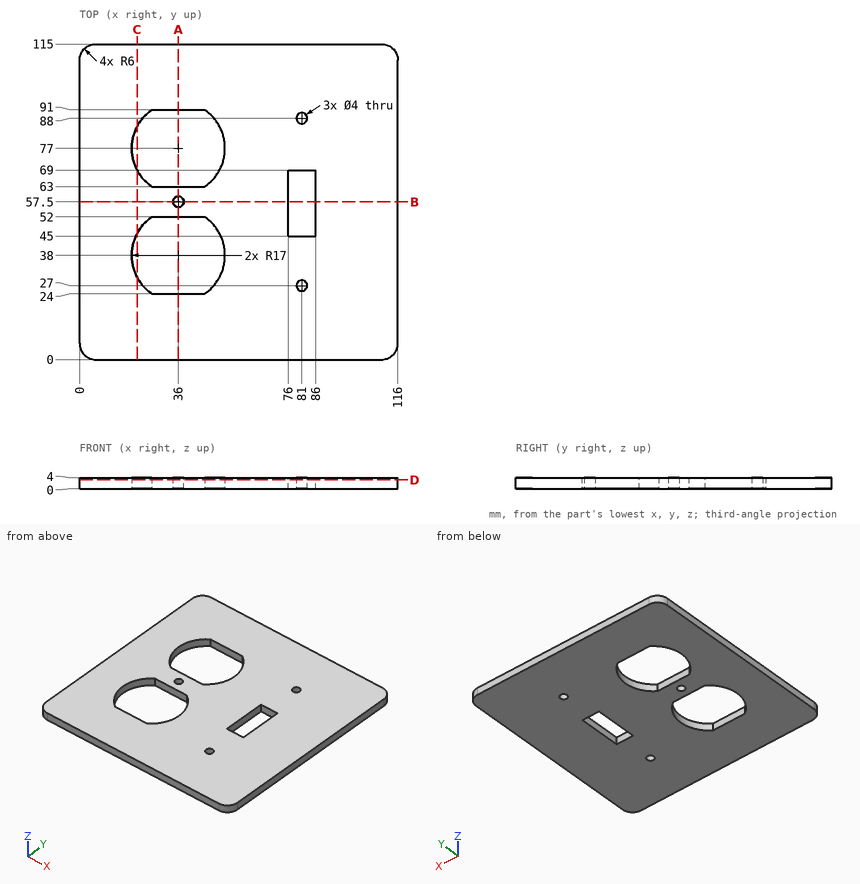
Design review of the part shown in the three views and the two pictorial views. Dimensions are in mm from the part's minimum x, y and z. Round coordinates to 2 decimals unless told otherwise and drop trailing zeros. Loops run counter-clockwise (first coordinate to the right, second up) from the corner with the lowest first, then second, coordinate; pieces in that order, holes last. Notation, with made-up numbers: M -6.5,3.25 L 42.5,3.25 A21 cw 42.5,26.25 Z; hole C -31,83.25 d8. An arc over 180 degrees is marked long. Put each result on its own line as item: value.
Q1. Consider section C-C, the plane x = 21. Give the boundary of the cut face in (y, z).
Result set:
outline: M 0,0 L 30,0 L 30,4 L 0,4 Z; M 46,0 L 69,0 L 69,4 L 46,4 Z; M 85,0 L 115,0 L 115,4 L 85,4 Z
Q2. Consider section D-D, the plane z = 3.2. Give the boundary of the cut face in (x, y), then the cut area to 3 significant figures.
Result set:
outline: M 0,6 A6 ccw 6,0 L 110,0 A6 ccw 116,6 L 116,109 A6 ccw 110,115 L 6,115 A6 ccw 0,109 Z; hole M 26.36,24 L 45.64,24 A17 ccw 45.64,52 L 26.36,52 A17 ccw Z; hole M 26.36,63 L 45.64,63 A17 ccw 45.64,91 L 26.36,91 A17 ccw Z; hole C 36,57.5 d4; hole M 76,45 L 86,45 L 86,69 L 76,69 Z; hole C 81,27 d4; hole C 81,88 d4
area: 11,400 mm²
Q3. Consider section B-B, the plane y = 57.5. Give the boundary of the cut face in (x, z), then the cut area to 3 significant figures.
Result set:
outline: M 0,0 L 34,0 L 34,4 L 0,4 Z; M 38,0 L 76,0 L 76,4 L 38,4 Z; M 86,0 L 116,0 L 116,4 L 86,4 Z
area: 408 mm²
Q4. To check wall thickness, follow L1, parallel to Y at x = 81, z = 1; L2, parallel to X at y = 57.5, z = 1.1; L3, parallel to Y at x = 36, z = 1.8. State the ranges of each line that lie inside material, in increasing order.
Result set:
L1: y = 0 to 25, 29 to 45, 69 to 86, 90 to 115
L2: x = 0 to 34, 38 to 76, 86 to 116
L3: y = 0 to 24, 52 to 55.5, 59.5 to 63, 91 to 115
Q5. For pin 1 (1.2 mm diameter, centred on x = 80.5, z = 1, fed in from -Y), flat-tipped, find the tip position at first contact; note if it passes through.
Result set:
pin 1: stops at y = 0
Q6. Consider section A-A, the plane x = 36. Give the boundary of the cut face in (y, z), then the cut area to 3 significant figures.
Result set:
outline: M 0,0 L 24,0 L 24,4 L 0,4 Z; M 52,0 L 55.5,0 L 55.5,4 L 52,4 Z; M 59.5,0 L 63,0 L 63,4 L 59.5,4 Z; M 91,0 L 115,0 L 115,4 L 91,4 Z
area: 220 mm²
